from build123d import *

# Parameters (mm, degrees)
SKETCH1_R               = 22.5
BOSS_EXTRUDE1_DEPTH     = 17.5
SKETCH2_R               = 17.5
CUT_EXTRUDE1_DEPTH      = 25
CUT_EXTRUDE2_DEPTH      = 37.314597616
CUT_EXTRUDE2_DEPTH_BACK = 37.314597616
SKETCH3_R               = 2.75
CUT_EXTRUDE3_DEPTH      = 37.314597788
CUT_EXTRUDE3_DEPTH_BACK = 37.314597788
SKETCH4_R               = 2.75
SKETCH5_R               = 1.75
CUT_EXTRUDE4_DEPTH      = 10


with BuildPart() as part:
    # Sketch1 → Boss-Extrude1 (new, symmetric)
    with BuildSketch(Plane(origin=(0, 0, 0), x_dir=(1, 0, 0), z_dir=(0, 1, 0))):
        with Locations(Location((0, 0, 0), (0, 0, 270))):
            Circle(SKETCH1_R)
    extrude(amount=BOSS_EXTRUDE1_DEPTH, both=True)

    # Sketch2 → Cut-Extrude1 (cut)
    with BuildSketch(Plane.XZ.offset(17.5)):
        with Locations(Location((0, 0, 0), (0, 0, 270))):
            Circle(SKETCH2_R)
    extrude(amount=-CUT_EXTRUDE1_DEPTH, mode=Mode.SUBTRACT)

    # Sketch3 → Cut-Extrude2 (cut, two sides: drawn at the far end of the back side and taken through both)
    with BuildSketch(Plane(origin=(0, 0, 0), x_dir=(0, 0, -1), z_dir=(1, 0, 0)).offset(-CUT_EXTRUDE2_DEPTH_BACK)):
        with Locations((0, -10)):
            Circle(SKETCH3_R)
    extrude(amount=CUT_EXTRUDE2_DEPTH + CUT_EXTRUDE2_DEPTH_BACK, mode=Mode.SUBTRACT)

    # Sketch4 → Cut-Extrude3 (cut, two sides: drawn at the far end of the back side and taken through both)
    with BuildSketch(Plane.XY.offset(-CUT_EXTRUDE3_DEPTH_BACK)):
        with Locations((0, -10)):
            Circle(SKETCH4_R)
    extrude(amount=CUT_EXTRUDE3_DEPTH + CUT_EXTRUDE3_DEPTH_BACK, mode=Mode.SUBTRACT)

    # Sketch5 → Cut-Extrude4 (cut)
    with BuildSketch(Plane(origin=(0, 17.5, 0), x_dir=(1, 0, 0), z_dir=(0, 1, 0))):
        with Locations(Location((0, 12.425, 0), (0, 0, 270))):
            Circle(SKETCH5_R)
        with Locations(Location((0, 8, 0), (0, 0, 270))):
            Circle(SKETCH5_R)
        with Locations(Location((0, -8, 0), (0, 0, 90))):
            Circle(SKETCH5_R)
        with Locations(Location((0, -12.425, 0), (0, 0, 90))):
            Circle(SKETCH5_R)
        with Locations(Location((-9.35, 0, 0), (0, 0, 270))):
            Circle(SKETCH5_R)
        with Locations(Location((9.35, 0, 0), (0, 0, 270))):
            Circle(SKETCH5_R)
    extrude(amount=-CUT_EXTRUDE4_DEPTH, mode=Mode.SUBTRACT)


solid = part.part
CAD build for the part. Positions are in the model's coordinates, mm. A direction names the side the tool comes from. Coordinates: 2 decimals unless noted, no trailing zeros. Write each loop counter-clockwise with the first axis right and the second up, starting at its lowest first coordinate (ties: lowest second). Pieces come first, ordered by that corner, then holes. Notation, with made-up numbers: M 61,80.25 L 109,80.25 A27 cw 109,108.25 Z; hole C 1,28.5 d1. An arc over 180 degrees is marked long. Return JSON: item names as keys, results as strings.
Item 1: Slice it at C-C, the plane z = 7.5. Write the cut outline in (x, y), and give its area (3 significant figures).
Findings below:
{"outline": "M -21.21,-17.5 L -15.81,-17.5 L -15.81,7.5 L -1.68,7.5 L -1.68,17.5 L -21.21,17.5 Z; M 1.68,7.5 L 15.81,7.5 L 15.81,-17.5 L 21.21,-17.5 L 21.21,17.5 L 1.68,17.5 Z", "area": "661 mm2"}
Item 2: Slice it at A-A, the plane x = 0. State how many separate pieces and enclosed holes the cut face has, and give its area (3 significant figures).
Findings below:
{"separate pieces": "7", "enclosed holes": "0", "area": "505 mm2"}
Item 3: Which spindle directions (+Z, -Z, +X, -X, +Y, -Y) get a long thin tool onto all of the face, cutting with end or side? Do faces 1 (the cylindrical face through (0.077, 12.57, -14.173)), 2 (the flat face through (0, 7.5, 0)). Say none if no direction does.
Findings below:
{"face 1": "+Y, -Y", "face 2": "-Y"}
Item 4: Two-plate mould, pull along Z, no slides. Class faces 3 (the cylindrical face through (-0.077, 12.57, 14.173)), 4 (the cylindrical face through (-2.027, -8.141, -19.93)), 5 (the cylindrical face through (6.76, 0.25, 21.46)): +Z half, -Z half, draft (parallel to the pull), parting line (faces both ways), or undercut.
Findings below:
{"face 3": "undercut", "face 4": "draft", "face 5": "parting line"}
Item 5: Probe line 1 (X direction, y = 10, z = 0); line 2 (Y direction, x = 19, z = 0); line 3 (X direction, y = 8, z = -1.5). List the from-to ranges inside material, lowest first. Write a range as from..to.
Findings below:
{"line 1": "x = -22.5..-11.1, -7.6..7.6, 11.1..22.5", "line 2": "y = -17.5..-12.75, -7.25..17.5", "line 3": "x = -22.45..-10.25, -8.45..8.45, 10.25..22.45"}
Item 6: Slice it at D-D, the plane x = 9.35. Write the cut outline in (y, z).
Findings below:
{"outline": "M -17.5,-20.47 L 17.5,-20.47 L 17.5,-1.75 L 7.5,-1.75 L 7.5,-14.79 L -17.5,-14.79 Z; M -17.5,14.79 L 7.5,14.79 L 7.5,1.75 L 17.5,1.75 L 17.5,20.47 L -17.5,20.47 Z"}
Item 7: Drop flat-ended pins along their axis: pin 1 Ø4.5 at (x, z) = (9.35, 0) entering from -Y; pin 2 Ø3 at (x, z) = (0, 12.425) entering from +Y; pin 3 Ø1 at (y, z) = (-11, 11) entering from +X; pin 4 Ø1.5 at (x, y) = (7, 3.5) entering from +Z. Give the stop position or say it passes through.
Findings below:
{"pin 1": "stops at y = 7.5", "pin 2": "passes through", "pin 3": "stops at x = 19.9", "pin 4": "stops at z = 21.61"}
Item 8: Slice it at B-B, the plane y = -10. Write the cut outline in (x, z).
Findings below:
{"outline": "M -22.33,-2.75 A22.5 ccw -2.75,-22.33 L -2.75,-17.28 A17.5 cw -17.28,-2.75 Z; M -22.33,2.75 L -17.28,2.75 A17.5 cw -2.75,17.28 L -2.75,22.33 A22.5 ccw Z; M 2.75,-22.33 A22.5 ccw 22.33,-2.75 L 17.28,-2.75 A17.5 cw 2.75,-17.28 Z; M 2.75,17.28 A17.5 cw 17.28,2.75 L 22.33,2.75 A22.5 ccw 2.75,22.33 Z"}
